```python
from build123d import *

# Parameters (mm, degrees)
CROQUIS2_W              = 50
CROQUIS2_H              = 150
SALIENTE_EXTRUIR1_DEPTH = 25
CROQUIS6_W              = 48
CROQUIS6_H              = 40
CORTAR_EXTRUIR1_DEPTH   = 25
VACIADO2_START          = -31.864905155
VACIADO2_OUTLINE_W      = 110
VACIADO2_OUTLINE_H      = 23
VACIADO2_DEPTH          = 48
CROQUIS8_R              = 4.5
CORTAR_EXTRUIR3_DEPTH   = 1
CROQUIS9_W              = 48
CROQUIS9_H              = 110
CORTAR_EXTRUIR4_DEPTH   = 10
CORTAR_EXTRUIR5_DEPTH   = 1
CORTAR_EXTRUIR6_DEPTH   = 1
CROQUIS12_R             = 1.5
CORTAR_EXTRUIR7_DEPTH   = 1
CROQUIS13_R             = 3
CORTAR_EXTRUIR8_DEPTH   = 10
REDONDEO1_R             = 10
CORTAR_EXTRUIR9_DEPTH   = 50


# Read off the part's stored shape, not the designer's step: Vaciado2
with BuildPart() as part:
    # Croquis2 → Saliente-Extruir1 (new body)
    with BuildSketch(Plane.XY):
        with Locations((-7.864905155, -22.416151752)):
            Rectangle(CROQUIS2_W, CROQUIS2_H)
    extrude(amount=SALIENTE_EXTRUIR1_DEPTH)

    # Croquis6 → Cortar-Extruir1 (cut)
    with BuildSketch(Plane(origin=(0, 0, 0), x_dir=(-1, 0, 0), z_dir=(0, 0, -1))):
        with Locations((7.864905155, 32.583848248)):
            Rectangle(CROQUIS6_W, CROQUIS6_H)
    extrude(amount=-CORTAR_EXTRUIR1_DEPTH, mode=Mode.SUBTRACT)

    # Vaciado2 outline → Vaciado2 (cut)
    with BuildSketch(Plane.YZ.offset(VACIADO2_START)):
        with Locations((-42.416151752, 12.5)):
            Rectangle(VACIADO2_OUTLINE_W, VACIADO2_OUTLINE_H)
    extrude(amount=VACIADO2_DEPTH, mode=Mode.SUBTRACT)

    # Croquis8 → Cortar-Extruir3 (cut)
    with BuildSketch(Plane.ZY.offset(32.864905155)):
        with Locations(Location((12.5, 22.583848248, 0), (0, 0, 270))):
            Circle(CROQUIS8_R)
    extrude(amount=-CORTAR_EXTRUIR3_DEPTH, mode=Mode.SUBTRACT)

    # Croquis9 → Cortar-Extruir4 (cut)
    with BuildSketch(Plane(origin=(0, 0, 0), x_dir=(-1, 0, 0), z_dir=(0, 0, -1))):
        with Locations((7.864905155, -42.416151752)):
            Rectangle(CROQUIS9_W, CROQUIS9_H)
    extrude(amount=-CORTAR_EXTRUIR4_DEPTH, mode=Mode.SUBTRACT)

    # Croquis10 → Cortar-Extruir5 (cut)
    with BuildSketch(Plane.ZY.offset(32.864905155)):
        Polygon((0, 0), (24, -12.416151752), (24, -97.416151752), (0, -97.416151752), align=None)
    extrude(amount=-CORTAR_EXTRUIR5_DEPTH, mode=Mode.SUBTRACT)

    # Croquis11 → Cortar-Extruir6 (cut)
    with BuildSketch(Plane(origin=(17.135094845, 0, 0), x_dir=(0, 0, -1), z_dir=(1, 0, 0))):
        Polygon((0, 0), (-24, -12.416151752), (-24, -97.416151752), (0, -97.416151752), align=None)
    extrude(amount=-CORTAR_EXTRUIR6_DEPTH, mode=Mode.SUBTRACT)

    # Croquis12 → Cortar-Extruir7 (cut)
    with BuildSketch(Plane(origin=(17.135094845, 0, 0), x_dir=(0, 0, -1), z_dir=(1, 0, 0))):
        with Locations(Location((-12.5, 22.583848248, 0), (0, 0, 90))):
            Circle(CROQUIS12_R)
    extrude(amount=-CORTAR_EXTRUIR7_DEPTH, mode=Mode.SUBTRACT)

    # Croquis13 → Cortar-Extruir8 (cut)
    with BuildSketch(Plane.XY.offset(25)):
        with Locations((-7.864905155, -22.248967482)):
            Circle(CROQUIS13_R)
        with BuildLine():
            Line((-17.864905155, -50.957171414), (-17.864905155, -70.930859048))
            ThreePointArc((-17.864905155, -70.930859048), (-17.791905055, -72.408923317), (-17.57361529, -73.872601075))
            Line((-17.57361529, -73.872601075), (-12.864905155, -97.416151752))
            Line((-12.864905155, -97.416151752), (-32.864905155, -97.416151752))
            Line((-32.864905155, -97.416151752), (-32.864905155, -17.416151752))
            Line((-32.864905155, -17.416151752), (-19.44849729, -44.248967482))
            ThreePointArc((-19.44849729, -44.248967482), (-18.266170313, -47.510877606), (-17.864905155, -50.957171414))
        make_face()
        Polygon((-27.864905155, -17.416151752), (-23.3927692, -15.180083774), (-10.976361335, -40.012899504), (-15.44849729, -42.248967482), align=None)
        with BuildLine():
            Line((-2.864905155, -97.416151752), (1.84380498, -73.872601075))
            ThreePointArc((1.84380498, -73.872601075), (2.062094745, -72.408923317), (2.135094845, -70.930859048))
            Line((2.135094845, -70.930859048), (2.135094845, -50.957171414))
            ThreePointArc((2.135094845, -50.957171414), (2.536360003, -47.510877606), (3.71868698, -44.248967482))
            Line((3.71868698, -44.248967482), (17.135094845, -17.416151752))
            Line((17.135094845, -17.416151752), (17.135094845, -97.416151752))
            Line((17.135094845, -97.416151752), (-2.864905155, -97.416151752))
        make_face()
        Polygon((12.135094845, -17.416151752), (-0.28131302, -42.248967482), (-4.753448975, -40.012899504), (7.66295889, -15.180083774), align=None)
        Polygon((-7.864905155, -42.248967482), (-5.285539059, -42.248967482), (-5.285539059, -85.512580171), (-7.864905155, -89.795904878), (-10.976361335, -85.512580171), (-10.709188819, -42.248967482), align=None)
    extrude(amount=-CORTAR_EXTRUIR8_DEPTH, mode=Mode.SUBTRACT)

    # Redondeo1
    redondeo1_edges = [part.edges().sort_by_distance(p)[0] for p in [
        (16.635094845, 52.583848248, 25),
        (-32.364905155, 52.583848248, 0),
        (-32.364905155, 52.583848248, 25),
        (16.635094845, 52.583848248, 0),
    ]]
    fillet(redondeo1_edges, radius=REDONDEO1_R)

    # Croquis14 → Cortar-Extruir9 (cut)
    with BuildSketch(Plane.ZY.offset(32.864905155)):
        with BuildLine():
            Line((0, 0), (9.235899895, 1.20073778))
            ThreePointArc((9.235899895, 1.20073778), (11.659366349, 0.915331151), (13.659135181, -0.483086245))
            Line((13.659135181, -0.483086245), (24, -12.416151752))
            Line((24, -12.416151752), (0, 0))
        make_face()
    extrude(amount=-CORTAR_EXTRUIR9_DEPTH, mode=Mode.SUBTRACT)


solid = part.part
```
Verification items for the finished model (mm, model axes). A direction names the side the tool comes from. Coordinates: 2 decimals unless noted, no trailing zeros. Write each loop counter-clockwise with the first axis right and the second up, starting at its lowest first coordinate (ties: lowest second). Pieces come first, ordered by that corner, then holes. Notation, with made-up numbers: (80, 13) - (92, 13) arc R5 cw to (92, 17) - close; hole circle Ø5 at (56.5, 38.5). An arc over 180 degrees is marked (long way). One line per question, with ' | ' between items. Start each with the question number.
1. Section check B-B (z = 4.5). Enter the section's corners in (x, y), plus the area to 3 significant figures.
2. Gauge pin test, flat ends, axial feed: P1, Ø4, axis at y = 22.58, z = 12.5, coming from the -X side; P2, Ø8, axis at x = -16.5, y = -12.5, coming from the -Z side; P3, Ø0.5, axis at y = -62.5, z = 24.5, coming from the -X side; P4, Ø5, axis at x = 4.5, y = -29, coming from the +Z side. Record the tip position at first contact, or that the pin passes through.
3. Material ranges on line 1 along X through (y, z) = (21, 4.75), recorded low to high.
4. Section check A-A (y = -30). Enter the section's corners in (x, z), plus the area to 3 significant figures.
5. Section check C-C (y = -48.5). Enter the section's corners in (x, z).
6. Draft check along X on faces 4 (the flat face through (-26.251, -30.645, 24.507)), 5 (the flat face through (-21.57, -30.01, 24.51)), 6 (the flat face through (16.63, -6.37, 18.76)). Enter one of: released by +X, released by -X, zero draft, split by the parting line, or undercut.
7. Access from +Z, -Z, +X, -X, +Y, -Y to the whole of each face (thin tool, end or side, straight path). Record for faces 1 (the flat face through (-17.271, -27.423, 24.507)), 2 (the cylindrical face through (-32.358, 49.732, 21.993)), 3 (the cylindrical face through (-32.37, 18.29, 13.85)).
Computed values:
1) outline: (-32.86, 0.59) - (-31.86, 0.59) - (-31.86, 50.94) - (-32.86, 50.94) - close; (16.14, 0.59) - (17.14, 0.59) - (17.14, 50.94) - (16.14, 50.94) - close | area: 101 mm²
2) P1: x = 16.14 | P2: z = 24 | P3: x = -17.86 | P4: z = 25
3) line 1: -32.86 to -31.86, 16.14 to 17.14
4) outline: (-26.57, 24) - (-21.57, 24) - (-21.57, 25) - (-26.57, 25) - close; (-15.98, 24) - (0.25, 24) - (0.25, 25) - (-15.98, 25) - close; (5.84, 24) - (10.84, 24) - (10.84, 25) - (5.84, 25) - close | area: 26.2 mm²
5) outline: (-18.07, 24) - (-10.75, 24) - (-10.75, 25) - (-18.07, 25) - close; (-5.29, 24) - (2.34, 24) - (2.34, 25) - (-5.29, 25) - close
6) face 4: released by -X | face 5: undercut | face 6: zero draft
7) face 1: +Z, -Z | face 2: +Z, +X, -X, +Y | face 3: -X
